Could you check a few things on this drawing? It's one solid part, dimensions in mm from its lowest x, y, z. Coordinates: 2 decimals unless noted, no trailing zeros. Loops run counter-clockwise (first coordinate to the right, second up) from the corner with the lowest first, then second, coordinate; pieces in that order, holes last.
1) Will these pins go through, and if not, where does the flat tip stop? P1, Ø4, axis at y = 9.5, z = 17, coming from the -X side; P2, Ø2, axis at x = 10, z = 20.5, coming from the -Y side; P3, Ø4, axis at x = 12.5, z = 19.5, coming from the -Y side; P4, Ø2, axis at x = 5.5, y = 7.5, coming from the +Z side.
2) If I drill on line 1 along Z through (x, y) = (4, 12.5); line 2 along Z through (x, y) = (10.5, 7); line 3 along Y through (x, z) = (1.25, 14.25), over which ranges is the centre line in solid material (lowest first)?
3) Thinking about a two-plate mould opening in Z: for the marked faces 1, 2 and 3, which applies, released by +Z, released by -Z, zero draft, split by the parting line, or undercut?
4) Imagine slicing it at C-C on x = 5.5. Please give me the cut outline in (y, z), plus the area to 3 significant figures.
5) Imagine slicing it at A-A on y = 12.5. Please give me the cut outline in (x, z), plus the area to 3 significant figures.
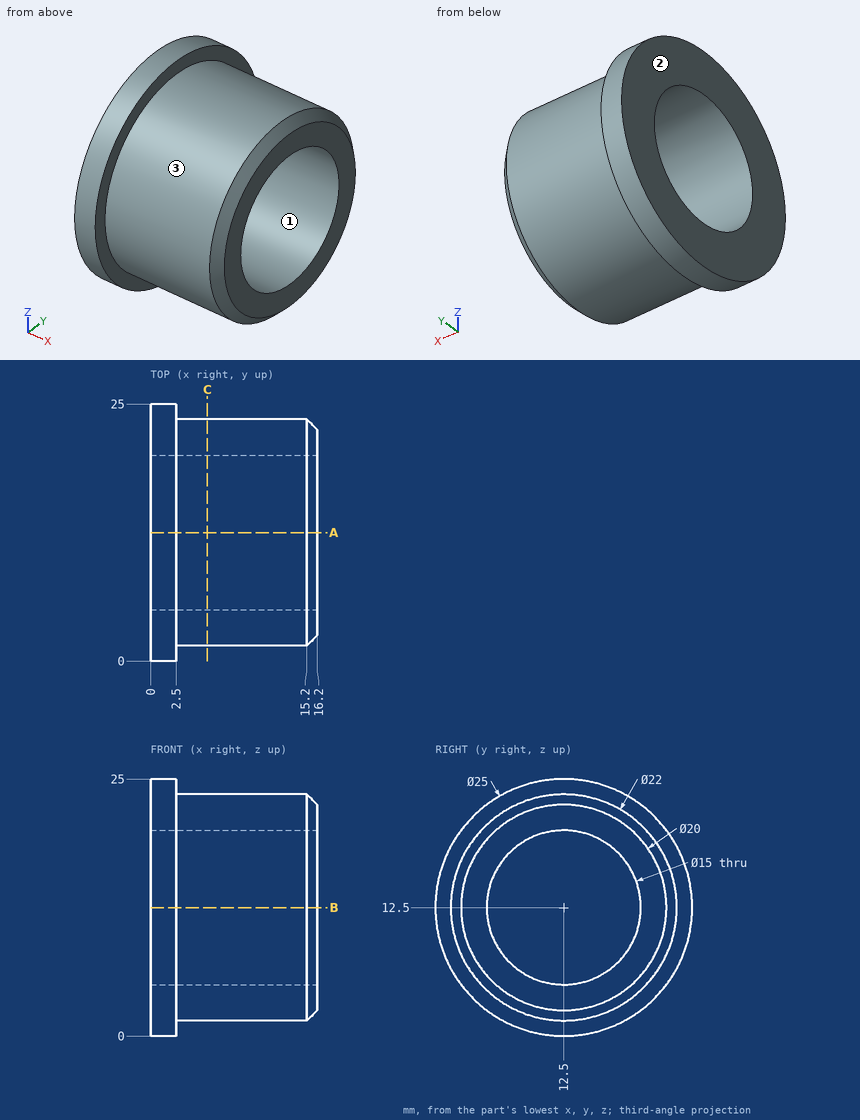
Filled in:
1. P1: passes through
1. P2: stops at y = 4.01
1. P3: stops at y = 2.7
1. P4: stops at z = 22.75
2. line 1: z = 1.5 to 5, 20 to 23.5
2. line 2: z = 2.97 to 7.4, 17.6 to 22.03
2. line 3: y = 0.12 to 5.21, 19.79 to 24.88
3. face 1: undercut
3. face 2: zero draft
3. face 3: split by the parting line
4. outline: circle Ø22 at (12.5, 12.5); hole circle Ø15 at (12.5, 12.5)
4. area: 203 mm2
5. outline: (0, 0) - (2.5, 0) - (2.5, 1.5) - (15.2, 1.5) - (16.2, 2.5) - (16.2, 5) - (0, 5) - close; (0, 20) - (16.2, 20) - (16.2, 22.5) - (15.2, 23.5) - (2.5, 23.5) - (2.5, 25) - (0, 25) - close
5. area: 120 mm2
